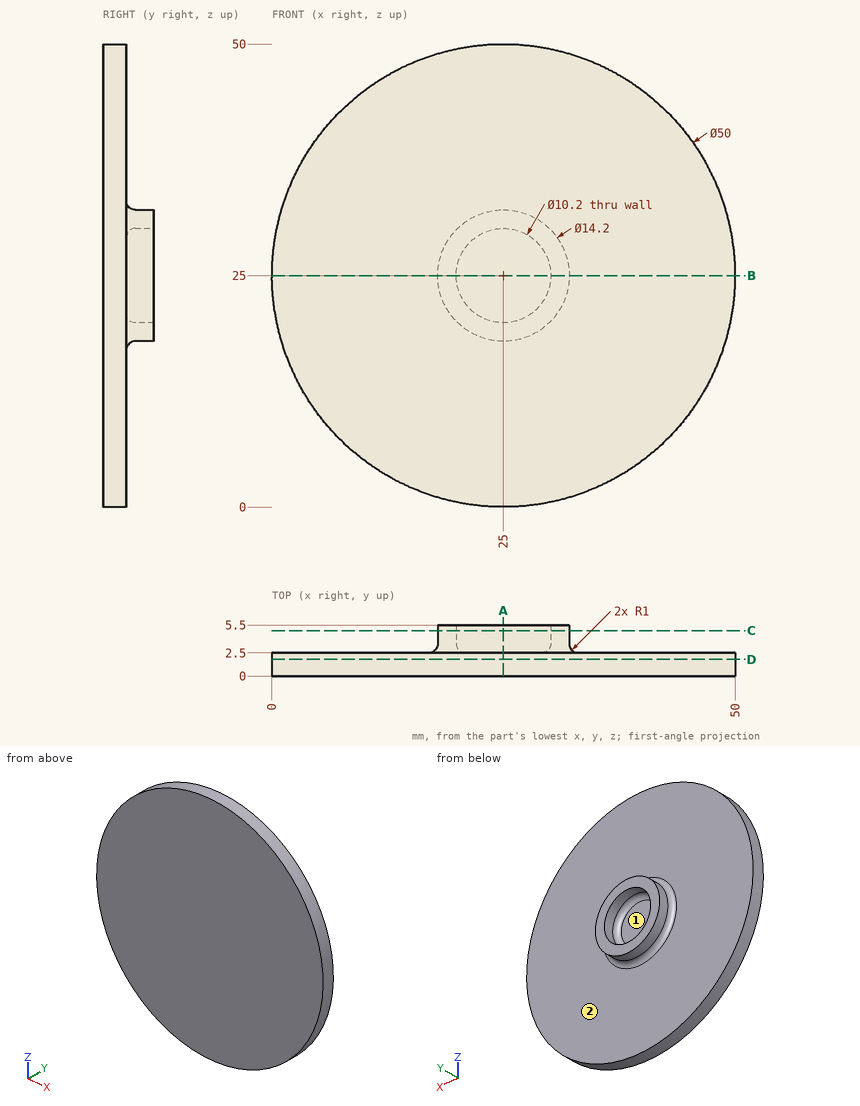
Geometry: see drawing. Coordinates: mm, zero at the bounding-box minimum. Give positions to 0.01 mm unless a question says otherwise; leave off trailing zeros. Order: outer loops, then holes, each group sorted by start corner. A loop starts at its lowest first (then second) coordinate and runs counter-clockwise, first axis right, second up.
Q1. Section D-D on y = 1.8. Output: boundary loops of the cut face in (x, z), and give its area (3 significant figures).
Checked values:
outline: circle Ø50 at (25, 25)
area: 1,960 mm2
Q2. Section A-A on x = 25. Output: boundary loops of the cut face in (y, z), and give its area (3 significant figures).
Checked values:
outline: (0, 0) - (2.5, 0) - (2.5, 16.9) arc R1 cw to (3.5, 17.9) - (5.5, 17.9) - (5.5, 19.9) - (3.5, 19.9) arc R1 cw to (2.5, 20.9) - (2.5, 29.1) arc R1 cw to (3.5, 30.1) - (5.5, 30.1) - (5.5, 32.1) - (3.5, 32.1) arc R1 cw to (2.5, 33.1) - (2.5, 50) - (0, 50) - close
area: 138 mm2
Q3. Draft query along Z for the marked faces 1 and 2. Return one class per face: +Z half, -Z half, draft (parallel to the pull), parting line (faces both ways), or undercut.
Checked values:
face 1: undercut
face 2: draft
Q4. Section C-C on y = 4.9. Output: boundary loops of the cut face in (x, z), and give its area (3 significant figures).
Checked values:
outline: circle Ø14.2 at (25, 25); hole circle Ø10.2 at (25, 25)
area: 76.7 mm2
Q5. Section B-B on z = 25. Output: boundary loops of the cut face in (x, y), and give its area (3 significant figures).
Checked values:
outline: (0, 0) - (50, 0) - (50, 2.5) - (33.1, 2.5) arc R1 cw to (32.1, 3.5) - (32.1, 5.5) - (30.1, 5.5) - (30.1, 3.5) arc R1 cw to (29.1, 2.5) - (20.9, 2.5) arc R1 cw to (19.9, 3.5) - (19.9, 5.5) - (17.9, 5.5) - (17.9, 3.5) arc R1 cw to (16.9, 2.5) - (0, 2.5) - close
area: 138 mm2
Q6. Ray query, probe 1 along X at (y, z) = (4.3, 25); probe 2 along Y at (x, z) = (15, 24.5); probe 3 along X at (y, z) = (2.9, 25.5). Return the intervals inside material, ascending.
Checked values:
probe 1: x = 17.9 to 19.9, 30.1 to 32.1
probe 2: y = 0 to 2.5
probe 3: x = 17.72 to 20.13, 29.87 to 32.28
Q7. Contact query for flat-ended pins moving along their axis: pin 1 Ø6.5 at (x, z) = (25, 25.5) entering from +Y; pin 2 Ø3 at (x, z) = (16, 23.5) entering from +Y; pin 3 Ø1 at (y, z) = (2, 43) entering from +X. Output: stop coordinate, or through.
Checked values:
pin 1: stops at y = 2.5
pin 2: stops at y = 2.62
pin 3: stops at x = 42.85
